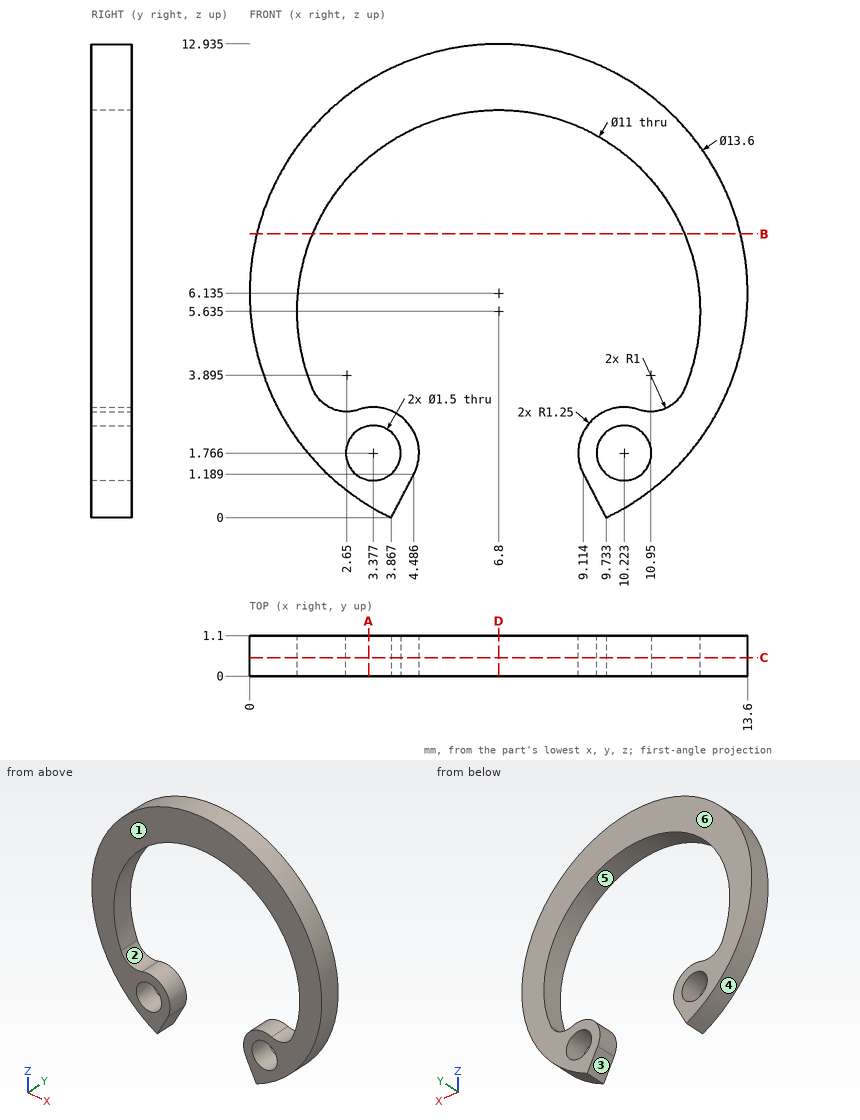
Part print with two shaded views. Sizes in mm from the minimum x, y, z corner. A direction names the side the tool comes from. Round coordinates to 2 decimals unless told otherwise and drop trailing zeros. Write each loop counter-clockwise with the first axis right and the second up, starting at its lowest first coordinate (ties: lowest second). Pieces come first, ordered by that corner, then holes. Notation, with made-up numbers: M 8.5,25 L 21.5,25 A23 ccw 21.5,54 Z; hole C 71.5,-9 d6. An arc over 180 degrees is marked long. Put each result on its own line as item: value. Start each with the question number.
1) Saw through at A-A, the plane x = 3.25. Write the cut outline in (y, z) (1 decimal).
2) Pin check, flat tip, straight feed: pin 1 Ø3 at (x, z) = (10, 8.5) entering from -Y. Stop position of the tip, or through.
3) Saw through at C-C, the plane y = 0.5. Count the separate pieces of the cut face and the enclosed holes in it.
4) Saw through at D-D, the plane x = 6.8. Write the cut outline in (y, z) (1 decimal).
5) Saw through at B-B, the plane z = 7.75. Write the cut outline in (x, y) (1 decimal).
6) 3-axis set-ups, long thin cutter, end or side, ignore diameter. For the marked faces 1 and 2: which of +Z, -Z, +X, -X, +Y, -Y reach the whole face in a straight line?
7) Drill centre lines: probe 1 along Z at (x, y) = (3, 0.1) (1 decimal); probe 2 along X at (y, z) = (0.95, 0.5) (1 decimal); probe 3 along X at (y, z) = (0.7, 1.5) (1 decimal). Where is each one in solid material? Low to high. Write a range as [from, to].
8) Pull direction Z, two halves, no side cores. Call the marked faces 3, 4, 5 and 6: pulls with the +Z half, pulls with the -Z half, needs draft (parallel to the pull), parting line crosses it, or undercut.
Resolved:
1. outline: M 0,0.3 L 1.1,0.3 L 1.1,1 L 0,1 Z; M 0,2.5 L 1.1,2.5 L 1.1,3 L 0,3 Z; M 0,9.8 L 1.1,9.8 L 1.1,11.9 L 0,11.9 Z
2. pin 1: y = 0
3. separate pieces: 1
3. enclosed holes: 2
4. outline: M 0,11.1 L 1.1,11.1 L 1.1,12.9 L 0,12.9 Z
5. outline: M 0.2,0 L 1.7,0 L 1.7,1.1 L 0.2,1.1 Z; M 11.9,0 L 13.4,0 L 13.4,1.1 L 11.9,1.1 Z
6. face 1: +Z, -Z, +X, -X, -Y
6. face 2: +Y, -Y
7. probe 1: [0.5, 1.1], [2.4, 3], [9.6, 11.8]
7. probe 2: [3, 4.1], [9.5, 10.6]
7. probe 3: [1.8, 2.7], [4.1, 4.6], [9, 9.5], [10.9, 11.8]
8. face 3: pulls with the -Z half
8. face 4: parting line crosses it
8. face 5: undercut
8. face 6: needs draft
